from build123d import *

# Parameters (mm, degrees)
SKETCH1_W           = 175
SKETCH1_H           = 150
BOSS_EXTRUDE1_DEPTH = 5
SKETCH3_R           = 15
SKETCH3_R_2         = 10
CUT_EXTRUDE1_DEPTH  = 5
SKETCH4_W           = 16
SKETCH4_H           = 35
CUT_EXTRUDE2_DEPTH  = 2
FILLET1_R           = 3


with BuildPart() as part:
    # Sketch1 → Boss-Extrude1 (new body)
    with BuildSketch(Plane.XY):
        with Locations((-87.5, -75)):
            Rectangle(SKETCH1_W, SKETCH1_H)
    extrude(amount=BOSS_EXTRUDE1_DEPTH)

    # Sketch3 → Cut-Extrude1 (cut)
    with BuildSketch(Plane.XY.offset(5)):
        with Locations((-30, -43)):
            Circle(SKETCH3_R)
        with Locations((-113, -43)):
            Circle(SKETCH3_R_2)
    extrude(amount=-CUT_EXTRUDE1_DEPTH, mode=Mode.SUBTRACT)

    # Sketch4 → Cut-Extrude2 (cut)
    with BuildSketch(Plane.XY.offset(5)):
        with Locations((-167, -17.5)):
            Rectangle(SKETCH4_W, SKETCH4_H)
        with Locations((-8, -17.5)):
            Rectangle(SKETCH4_W, SKETCH4_H)
        with Locations((-8, -132.5)):
            Rectangle(SKETCH4_W, SKETCH4_H)
        with Locations((-167, -132.5)):
            Rectangle(SKETCH4_W, SKETCH4_H)
    extrude(amount=-CUT_EXTRUDE2_DEPTH, mode=Mode.SUBTRACT)

    # Fillet1
    fillet1_edges = [part.edges().sort_by_distance(p)[0] for p in [
        (0, -150, 1.5),
        (-175, -150, 1.5),
        (-175, 0, 1.5),
        (0, 0, 1.5),
    ]]
    fillet(fillet1_edges, radius=FILLET1_R)


solid = part.part
Input: part model. Units: mm. Frame: model coordinates. A direction names the side the tool comes from. Coordinates: 2 decimals unless noted, no trailing zeros. Loops run counter-clockwise (first coordinate to the right, second up) from the corner with the lowest first, then second, coordinate; pieces in that order, holes last. Notation, with made-up numbers: (35.25, 7) - (94.25, 7) arc R31 ccw to (94.25, 44) - close; hole circle Ø7 at (49, 68.25). An arc over 180 degrees is marked (long way). Answer in a Markdown table with one row per item. Add a question column.
Item 1: Line query: line 1 along Y through (x, z) = (-113, 2.4); line 2 along X through (y, z) = (-38, 0.3); line 3 along Y through (x, z) = (-30, 1.5). Output: solid intervals per line, ascending. Write a range as [from, to].
Item 2: Section query B-B on x = -121. Return the cut outline in (y, z), then the cut area to 3 significant figures.
Item 3: Section query C-C on z = 0.85. Return the cut outline in (x, y).
Item 4: Section query A-A on y = -43. Return the cut outline in (x, z).
Item 5: Mould query, pull axis X, two halves, no side actions, for faces 1 (the flat face through (-8, -132, 3)), 2 (the cylindrical face through (-115.17, -52.76, 2.54)), 3 (the flat face through (-175, -76, 2)). Classes: released by +X, released by -X, zero draft, split by the parting line, or undercut.
Item 6: Contact query for flat-ended pins moving along their axis: P1, Ø5, axis at x = -171, y = -135.5, coming from the +Z side; P2, Ø1, axis at y = -139, z = 4, coming from the -X side; P3, Ø1.6, axis at x = -8.5, z = 4.5, coming from the +Y side. Output: stop coordinate, or through.
Item 7: Access query for faces 4 (the flat face through (-89, -150, 2)), 5 (the flat face through (-167, -17, 3)), 6 (the flat face through (-167, -132, 3)), 7 (the flat face through (-89, -74, 5)), 8 (the flat face through (-8, -17, 3)). Directions: +Z, -Z, +X, -X, +Y, -Y. A direction counts if a zero-diameter tool reaches every point of the face in a straight line with its end or side. Return the directions, or none.
Item 8: Section query D-D on y = -126. Return the cut outline in (x, z).
Recorded:
| question | item | result |
|---|---|---|
| 1 | line 1 | [-150, -53], [-33, 0] |
| 1 | line 2 | [-175, -121.66], [-104.34, -44.14], [-15.86, 0] |
| 1 | line 3 | [-150, -58], [-28, 0] |
| 2 | outline | (-150, 0) - (-49, 0) - (-49, 5) - (-150, 5) - close; (-37, 0) - (0, 0) - (0, 5) - (-37, 5) - close |
| 2 | area | 690 mm^2 |
| 3 | outline | (-175, -147) arc R3 ccw to (-172, -150) - (-3, -150) arc R3 ccw to (0, -147) - (0, -3) arc R3 ccw to (-3, 0) - (-172, 0) arc R3 ccw to (-175, -3) - close; hole circle Ø20 at (-113, -43); hole circle Ø30 at (-30, -43) |
| 4 | outline | (-175, 0) - (-123, 0) - (-123, 5) - (-175, 5) - close; (-103, 0) - (-45, 0) - (-45, 5) - (-103, 5) - close; (-15, 0) - (0, 0) - (0, 5) - (-15, 5) - close |
| 5 | face 1 | zero draft |
| 5 | face 2 | undercut |
| 5 | face 3 | released by -X |
| 6 | P1 | z = 3 |
| 6 | P2 | x = -159 |
| 6 | P3 | y = -35 |
| 7 | face 4 | +Z, -Z, +X, -X, -Y |
| 7 | face 5 | +Z, -X, +Y |
| 7 | face 6 | +Z, -X, -Y |
| 7 | face 7 | +Z, +X, -X, +Y, -Y |
| 7 | face 8 | +Z, +X, +Y |
| 8 | outline | (-175, 0) - (0, 0) - (0, 3) - (-16, 3) - (-16, 5) - (-159, 5) - (-159, 3) - (-175, 3) - close |
